Verification items for this drawing (mm, ordinates from the low corner). A direction names the side the tool comes from. Round coordinates to 2 decimals unless told otherwise and drop trailing zeros. Order: outer loops, then holes, each group sorted by start corner. A loop starts at its lowest first (then second) coordinate and runs counter-clockwise, first axis right, second up. Notation, with made-up numbers: (30.25, 44.25) -> (88.25, 44.25) arc R31 cw to (88.25, 75.25) -> close; hole circle Ø9 at (-34.5, 88.25). An arc over 180 degrees is marked (long way). Return JSON: item names as keys, results as strings. Group by question number.
Item 1: Sectioned sample at D-D on x = 16. Record the cut outline in (y, z).
Item 2: Access from +Z, -Z, +X, -X, +Y, -Y to the whole of each face (thin tool, end or side, straight path). Record for the marked faces 1, 2 and 3.
Item 3: Sectioned sample at B-B on y = 4.5. Record the cut outline in (x, z), plus the area to 3 significant figures.
Item 4: Sectioned sample at A-A on x = 4.5. Record the cut outline in (y, z).
Item 5: Depth check by flat-ended pin: pin 1 Ø1 at (x, z) = (4, 6) entering from +Y; pin 2 Ø3 at (y, z) = (4.5, 3) entering from -X; pin 3 Ø0.9 at (x, z) = (12, 2) entering from -Y; pin 4 Ø2 at (x, y) = (5.5, 22.5) entering from +Z. Enter the tip coordinate at first touch or a pass-through.
Item 6: Draft check along Y on the marked faces 4, 5 and 6. Enter one of: pulls with the +Y half, pulls with the -Y half, needs draft (parallel to the pull), parting line crosses it, or undercut.
Item 7: Scan lines: probe 1 along Z at (x, y) = (27.6, 4.5); probe 2 along Y at (x, z) = (25.5, 1.7); probe 3 along Y at (x, z) = (25.5, 2.4). Record each from-to range of solid material in increasing order. Write a range as from..to.
Item 8: Sectioned sample at C-C on z = 2. Record the cut outline in (x, y).
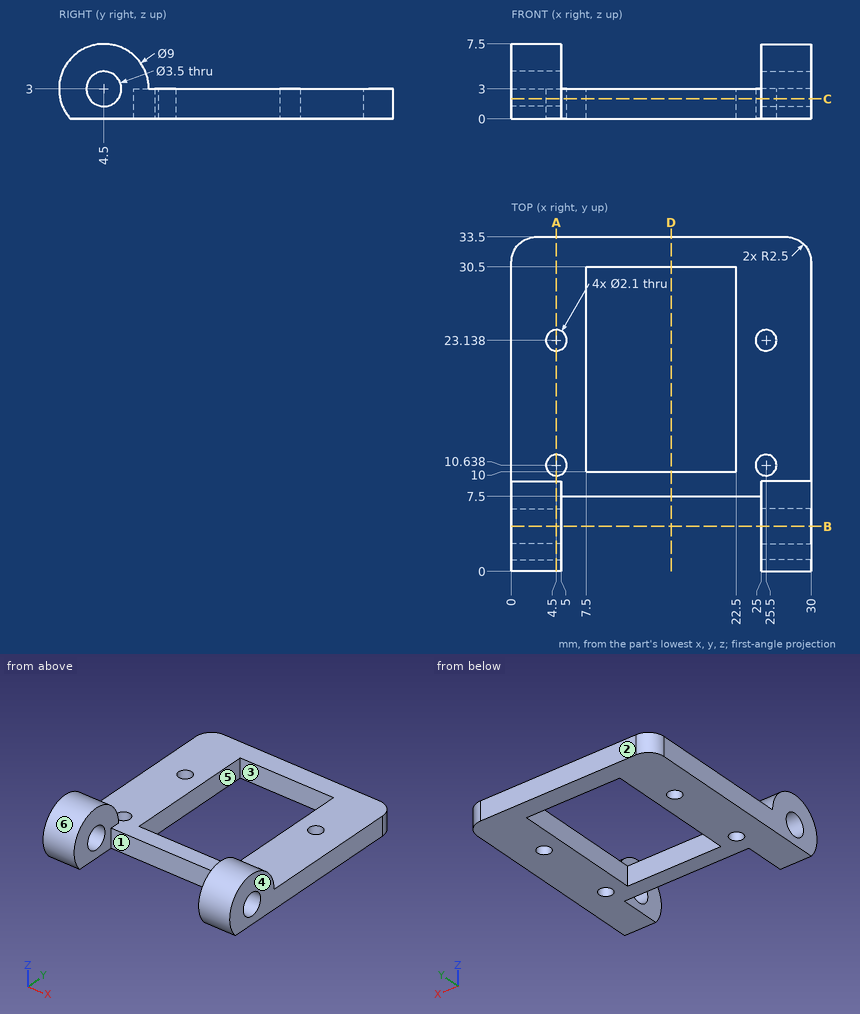
Recorded:
{
 "1": {"outline": "(7.5, 0) -> (10, 0) -> (10, 3) -> (7.5, 3) -> close; (30.5, 0) -> (33.5, 0) -> (33.5, 3) -> (30.5, 3) -> close"},
 "2": {"face 1": "+Z, -Z, -Y", "face 2": "+Z, -Z, +X, -X, +Y", "face 3": "+Z, -Z"},
 "3": {"outline": "(0, 0) -> (5, 0) -> (5, 1.25) -> (0, 1.25) -> close; (0, 4.75) -> (5, 4.75) -> (5, 7.5) -> (0, 7.5) -> close; (25, 0) -> (30, 0) -> (30, 1.25) -> (25, 1.25) -> close; (25, 4.75) -> (30, 4.75) -> (30, 7.5) -> (25, 7.5) -> close", "area": "40.0 mm²"},
 "4": {"outline": "(1.15, 0) -> (9.59, 0) -> (9.59, 3) -> (9, 3) arc R4.5 ccw (long way) to start; (11.69, 0) -> (22.09, 0) -> (22.09, 3) -> (11.69, 3) -> close; (24.19, 0) -> (33.5, 0) -> (33.5, 3) -> (24.19, 3) -> close; hole circle Ø3.5 at (4.5, 3)"},
 "5": {"pin 1": "y = 8.24", "pin 2": "through", "pin 3": "y = 7.5", "pin 4": "z = 3"},
 "6": {"face 4": "needs draft", "face 5": "undercut", "face 6": "parting line crosses it"},
 "7": {"probe 1": "0..1.25, 4.75..7.5", "probe 2": "0.19..3.33, 5.67..9.59, 11.69..22.09, 24.19..33.5", "probe 3": "0.04..2.86, 6.14..9.59, 11.69..22.09, 24.19..33.5"},
 "8": {"outline": "(0, 0.11) -> (5, 0.11) -> (5, 3.06) -> (0, 3.06) -> close; (0, 5.94) -> (5, 5.94) -> (5, 7.5) -> (25, 7.5) -> (25, 5.94) -> (30, 5.94) -> (30, 31) arc R2.5 ccw to (27.5, 33.5) -> (2.5, 33.5) arc R2.5 ccw to (0, 31) -> close; (25, 0.11) -> (30, 0.11) -> (30, 3.06) -> (25, 3.06) -> close; hole circle Ø2.1 at (4.5, 10.64); hole circle Ø2.1 at (4.5, 23.14); hole (7.5, 10) -> (22.5, 10) -> (22.5, 30.5) -> (7.5, 30.5) -> close; hole circle Ø2.1 at (25.5, 10.64); hole circle Ø2.1 at (25.5, 23.14)"}
}
